Build history of the part. All positions in model axes, mm. Coordinates: 2 decimals unless noted, no trailing zeros. Loops run counter-clockwise (first coordinate to the right, second up) from the corner with the lowest first, then second, coordinate; pieces in that order, holes last.
(1) Slice it at C-C (z = 17.7). Give the cut face in (x, y), and give its area (3 significant figures).
(2) Wall check: L1, parallel to Z at x = -5, y = -1.15; L2, parallel to X at y = 0.9, z = -63; L3, parallel to X at y = 0.7, z = 17.7. Give the ranges that are in metal, low to high.
(3) Slice it at A-A (y = -0.7). Give the cut face in (x, z), and give its area (3 significant figures).
(4) Slice it at B-B (x = 5). Give the cut face in (y, z), and give its area (3 significant figures).
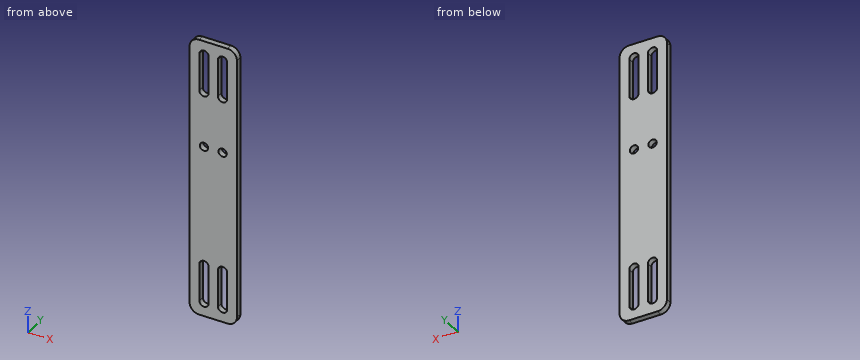
from build123d import *

# Parameters (mm, degrees)
BOSS_EXTRUDE1_DEPTH      = 76.2
BOSS_EXTRUDE1_DEPTH_BACK = 76.2
SKETCH3_W                = 25.4
SKETCH3_H                = 3.175
CUT_EXTRUDE2_DEPTH       = 3.175
FILLET1_R                = 5
M4_CLEARANCE_HOLE1_D     = 4.5


with BuildPart() as part:
    # Sketch3 → Boss-Extrude1 (new, two sides: drawn at the far end of the back side and taken through both)
    with BuildSketch(Plane.XY.offset(-BOSS_EXTRUDE1_DEPTH_BACK)):
        Rectangle(SKETCH3_W, SKETCH3_H)
    extrude(amount=BOSS_EXTRUDE1_DEPTH + BOSS_EXTRUDE1_DEPTH_BACK)

    # Sketch5 → Cut-Extrude2 (cut)
    with BuildSketch(Plane(origin=(0, -1.5875, 0), x_dir=(-1, 0, 0), z_dir=(0, -1, 0))):
        with BuildLine():
            Line((7.5, -48.1), (7.5, -68.5))
            ThreePointArc((7.5, -68.5), (5, -71), (2.5, -68.5))
            Line((2.5, -68.5), (2.5, -48.1))
            ThreePointArc((2.5, -48.1), (5, -45.6), (7.5, -48.1))
        make_face()
        with BuildLine():
            Line((-2.5, -48.1), (-2.5, -68.5))
            ThreePointArc((-2.5, -68.5), (-5, -71), (-7.5, -68.5))
            Line((-7.5, -68.5), (-7.5, -48.1))
            ThreePointArc((-7.5, -48.1), (-5, -45.6), (-2.5, -48.1))
        make_face()
    cut_extrude2 = extrude(amount=-CUT_EXTRUDE2_DEPTH, mode=Mode.SUBTRACT)

    # Mirror1: Cut-Extrude2 across plane
    add(cut_extrude2.mirror(Plane.XY), mode=Mode.SUBTRACT)

    # Fillet1
    fillet1_edges = [part.edges().sort_by_distance(p)[0] for p in [
        (12.7, 0, 76.2),
        (-12.7, 0, -76.2),
        (12.7, 0, -76.2),
        (-12.7, 0, 76.2),
    ]]
    fillet(fillet1_edges, radius=FILLET1_R)

    # M4 Clearance Hole1 (through all)
    with Locations(Plane(origin=(0, 1.5875, 0), x_dir=(1, 0, 0), z_dir=(0, 1, 0))):
        with Locations((5, -17.7), (-5, -17.7)):
            Hole(M4_CLEARANCE_HOLE1_D / 2)


solid = part.part
Response values:
1. outline: (-12.7, -1.59) - (-7.25, -1.59) - (-7.25, 1.59) - (-12.7, 1.59) - close; (-2.75, -1.59) - (2.75, -1.59) - (2.75, 1.59) - (-2.75, 1.59) - close; (7.25, -1.59) - (12.7, -1.59) - (12.7, 1.59) - (7.25, 1.59) - close
1. area: 52.1 mm2
2. L1: z = -76.2 to -71, -45.6 to 15.45, 19.95 to 45.6, 71 to 76.2
2. L2: x = -12.7 to -7.5, -2.5 to 2.5, 7.5 to 12.7
2. L3: x = -12.7 to -7.25, -2.75 to 2.75, 7.25 to 12.7
3. outline: (-12.7, -71.2) arc R5 ccw to (-7.7, -76.2) - (7.7, -76.2) arc R5 ccw to (12.7, -71.2) - (12.7, 71.2) arc R5 ccw to (7.7, 76.2) - (-7.7, 76.2) arc R5 ccw to (-12.7, 71.2) - close; hole (-7.5, -68.5) arc R2.5 ccw to (-2.5, -68.5) - (-2.5, -48.1) arc R2.5 ccw to (-7.5, -48.1) - close; hole (-7.5, 48.1) arc R2.5 ccw to (-2.5, 48.1) - (-2.5, 68.5) arc R2.5 ccw to (-7.5, 68.5) - close; hole circle Ø4.5 at (-5, 17.7); hole (2.5, -68.5) arc R2.5 ccw to (7.5, -68.5) - (7.5, -48.1) arc R2.5 ccw to (2.5, -48.1) - close; hole (2.5, 48.1) arc R2.5 ccw to (7.5, 48.1) - (7.5, 68.5) arc R2.5 ccw to (2.5, 68.5) - close; hole circle Ø4.5 at (5, 17.7)
3. area: 3,330 mm2
4. outline: (-1.59, -76.2) - (1.59, -76.2) - (1.59, -71) - (-1.59, -71) - close; (-1.59, -45.6) - (1.59, -45.6) - (1.59, 15.45) - (-1.59, 15.45) - close; (-1.59, 19.95) - (1.59, 19.95) - (1.59, 45.6) - (-1.59, 45.6) - close; (-1.59, 71) - (1.59, 71) - (1.59, 76.2) - (-1.59, 76.2) - close
4. area: 308 mm2
